The figure shows three views and two pictorial views of one solid part (mm, origin at its lowest corner). Answer the questions. A direction names the side the tool comes from. Round coordinates to 2 decimals unless told otherwise and drop trailing zeros. Write each loop counter-clockwise with the first axis right and the second up, starting at its lowest first coordinate (ties: lowest second). Pieces come first, ordered by that corner, then holes. Notation, with made-up numbers: (-4, 26) -> (23, 26) arc R25 cw to (23, 53) -> close; hole circle Ø10 at (-27, -5.75). An arc over 180 degrees is marked (long way). One line per item, written item: value.
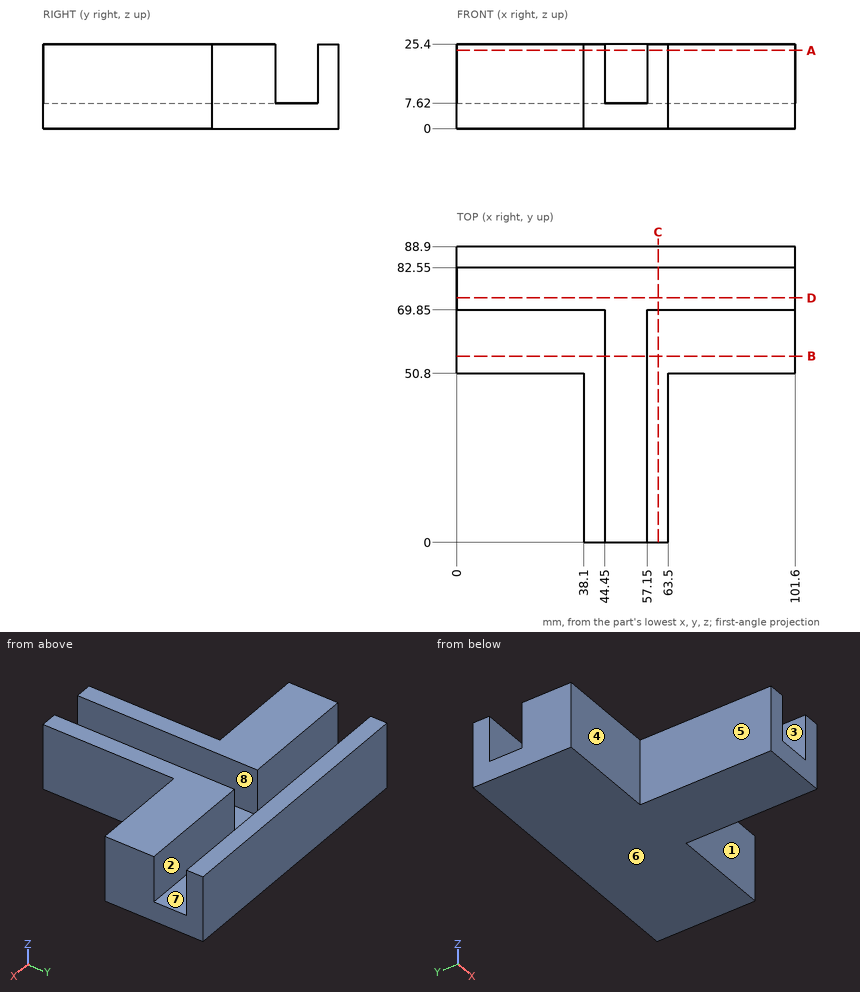
(1) Find section C-C on x = 60.5. Give the vertices of the cut face in (y, z).
Reported:
outline: (0, 0) -> (88.9, 0) -> (88.9, 25.4) -> (82.55, 25.4) -> (82.55, 7.62) -> (69.85, 7.62) -> (69.85, 25.4) -> (0, 25.4) -> close
(2) Find section D-D on y = 73.5. Give the vertices of the cut face in (x, z), plus the area to 3 significant figures.
Reported:
outline: (0, 0) -> (101.6, 0) -> (101.6, 7.62) -> (0, 7.62) -> close
area: 774 mm2
(3) A tool of negligible diameter and unlimited length cuts with its end or side. For the marked faces 1, 2, 3 and 4, from which of +Z, -Z, +X, -X, +Y, -Y can it reach the whole face along a straight path? Write none if from no direction.
Reported:
face 1: +Z, -Z, +X, -Y
face 2: +Z, +X, -X
face 3: +Z, -Y
face 4: +Z, -Z, -X, -Y
(4) For a pull along X with two mould halves and no side action, classify the marked faces 5, 6, 7 and 8 as pulls with the +X half, pulls with the -X half, needs draft (parallel to the pull), parting line crosses it, or undercut.
Reported:
face 5: pulls with the -X half
face 6: needs draft
face 7: undercut
face 8: undercut
(5) Find section B-B on y = 56. Give the vertices of the cut face in (x, z).
Reported:
outline: (0, 0) -> (101.6, 0) -> (101.6, 25.4) -> (57.15, 25.4) -> (57.15, 7.62) -> (44.45, 7.62) -> (44.45, 25.4) -> (0, 25.4) -> close
(6) Find section A-A on z = 23.5. Give the vertices of the cut face in (x, y), plus the area to 3 significant figures.
Reported:
outline: (0, 50.8) -> (38.1, 50.8) -> (38.1, 0) -> (44.45, 0) -> (44.45, 69.85) -> (0, 69.85) -> close; (0, 82.55) -> (101.6, 82.55) -> (101.6, 88.9) -> (0, 88.9) -> close; (57.15, 0) -> (63.5, 0) -> (63.5, 50.8) -> (101.6, 50.8) -> (101.6, 69.85) -> (57.15, 69.85) -> close
area: 2,980 mm2
(7) Consider probe 1 along X at (y, z) = (52.5, 16.5); probe 2 along Y at (x, z) = (71, 18); probe 3 along X at (y, z) = (47, 17.75). Determine where each line is inside the solid, lowest interval first.
Reported:
probe 1: x = 0 to 44.45, 57.15 to 101.6
probe 2: y = 50.8 to 69.85, 82.55 to 88.9
probe 3: x = 38.1 to 44.45, 57.15 to 63.5
(8) Flat-ended cylindrical pins translate along their axes: pin 1 Ø1 at (x, z) = (55.5, 12.5) entering from -Y; pin 2 Ø1.5 at (y, z) = (36, 11) entering from -X; pin 3 Ø2 at (y, z) = (34, 14) entering from +X. Find the tip coordinate at first contact, or state that the pin passes through.
Reported:
pin 1: stops at y = 82.55
pin 2: stops at x = 38.1
pin 3: stops at x = 63.5
